from build123d import *

# Parameters (mm, degrees)
SKETCH1_R            = 12.5
BOSS_EXTRUDE1_DEPTH  = 4
BOSS_EXTRUDE7_DEPTH  = 4
SKETCH9_W            = 20
SKETCH9_H            = 36
BOSS_EXTRUDE8_DEPTH  = 4
BOSS_EXTRUDE9_DEPTH  = 8
BOSS_EXTRUDE10_DEPTH = 4
FILLET4_R            = 1
SKETCH11_R           = 2.5
CUT_EXTRUDE2_DEPTH   = 57.25989309
CHAMFER1_SIZE        = 10
SKETCH12_R           = 2.5
CUT_EXTRUDE3_DEPTH   = 4
FILLET5_R            = 1
SCALE1_SCALE         = 0.5


with BuildPart() as part:
    # Sketch1 → Boss-Extrude1 (new body)
    with BuildSketch(Plane.XY):
        Circle(SKETCH1_R)
        with BuildLine():
            Line((26.387505004, 12.5), (20, 12.5))
            Line((20, 12.5), (20, -12.5))
            Line((20, -12.5), (26.387505004, -12.5))
            ThreePointArc((26.387505004, -12.5), (22, 0), (26.387505004, 12.5))
        make_face()
        with BuildLine():
            Line((13.612494996, 12.5), (0, 12.5))
            ThreePointArc((0, 12.5), (8.838834765, 8.838834765), (12.5, 0))
            ThreePointArc((12.5, 0), (8.838834765, -8.838834765), (0, -12.5))
            Line((0, -12.5), (13.612494996, -12.5))
            ThreePointArc((13.612494996, -12.5), (18, 0), (13.612494996, 12.5))
        make_face()
        with BuildLine():
            Line((20, 12.5), (13.612494996, 12.5))
            ThreePointArc((13.612494996, 12.5), (18, 0), (13.612494996, -12.5))
            Line((13.612494996, -12.5), (20, -12.5))
            Line((20, -12.5), (20, 12.5))
        make_face()
    extrude(amount=BOSS_EXTRUDE1_DEPTH)

    # Sketch8 → Boss-Extrude7 (add)
    with BuildSketch(Plane(origin=(0, 0, 0), x_dir=(-1, 0, 0), z_dir=(0, 0, -1))):
        with BuildLine():
            Line((-26.387505004, 12.5), (-41.387505004, 12.5))
            Line((-41.387505004, 12.5), (-41.387505004, -12.5))
            Line((-41.387505004, -12.5), (-26.387505004, -12.5))
            ThreePointArc((-26.387505004, -12.5), (-22, 0), (-26.387505004, 12.5))
        make_face()
    extrude(amount=-BOSS_EXTRUDE7_DEPTH)


with BuildPart() as body_2:
    # Mirror3: mirrored copy
    add(part.part.mirror(Plane.XY.offset(18)))


with BuildPart() as part_1:
    add(part.part)

    add(body_2.part)  # Boss-Extrude8 merges body 2
    # Sketch9 → Boss-Extrude8 (add)
    with BuildSketch(Plane.XZ.offset(12.5)):
        with Locations((31.387505004, 18)):
            Rectangle(SKETCH9_W, SKETCH9_H)
    extrude(amount=-BOSS_EXTRUDE8_DEPTH)

    # Sketch1_4 → Boss-Extrude9 (add)
    with BuildSketch(Plane.XY):
        with BuildLine():
            Line((20, 12.5), (13.612494996, 12.5))
            ThreePointArc((13.612494996, 12.5), (18, 0), (13.612494996, -12.5))
            Line((13.612494996, -12.5), (20, -12.5))
            Line((20, -12.5), (20, 12.5))
        make_face()
        with BuildLine():
            Line((26.387505004, 12.5), (20, 12.5))
            Line((20, 12.5), (20, -12.5))
            Line((20, -12.5), (26.387505004, -12.5))
            ThreePointArc((26.387505004, -12.5), (22, 0), (26.387505004, 12.5))
        make_face()
        with BuildLine():
            Line((40, 12.5), (26.387505004, 12.5))
            ThreePointArc((26.387505004, 12.5), (22, 0), (26.387505004, -12.5))
            Line((26.387505004, -12.5), (40, -12.5))
            ThreePointArc((40, -12.5), (27.5, 0), (40, 12.5))
        make_face()
    boss_extrude9 = extrude(amount=BOSS_EXTRUDE9_DEPTH)

    # Sketch10 → Boss-Extrude10 (add)
    with BuildSketch(Plane.XY.offset(4)):
        with BuildLine():
            Line((41.387505004, 12.5), (40, 12.5))
            ThreePointArc((40, 12.5), (28.543560763, 5), (30.83484861, -8.5))
            Line((30.83484861, -8.5), (41.387505004, -8.5))
            Line((41.387505004, -8.5), (41.387505004, 12.5))
        make_face()
    boss_extrude10 = extrude(amount=BOSS_EXTRUDE10_DEPTH)

    # Mirror4: Boss-Extrude9, Boss-Extrude10 across plane
    add(boss_extrude9.mirror(Plane.XY.offset(18)))
    add(boss_extrude10.mirror(Plane.XY.offset(18)))

    # Fillet4
    fillet4_edges = [part_1.edges().sort_by_distance(p)[0] for p in [
        (13.612494996, -12.5, 30),
        (13.612494996, 12.5, 30),
        (13.612494996, -12.5, 6),
        (13.612494996, 12.5, 6),
    ]]
    fillet(fillet4_edges, radius=FILLET4_R)

    # Sketch11 → Cut-Extrude2 (cut, through all)
    with BuildSketch(Plane.XY.offset(36)):
        Circle(SKETCH11_R)
    extrude(amount=-CUT_EXTRUDE2_DEPTH, mode=Mode.SUBTRACT)

    # Chamfer1
    chamfer1_edges = [part_1.edges().sort_by_distance(p)[0] for p in [
        (41.387505004, 12.5, 4),
        (41.387505004, 12.5, 32),
    ]]
    chamfer(chamfer1_edges, length=CHAMFER1_SIZE)

    # Sketch12 → Cut-Extrude3 (cut)
    with BuildSketch(Plane(origin=(0, -8.5, 0), x_dir=(1, 0, 0), z_dir=(0, 1, 0))):
        with Locations(Location((32.387505004, -12, 0), (0, 0, 180))):
            Circle(SKETCH12_R)
        with Locations((32.387505004, -24)):
            Circle(SKETCH12_R)
    extrude(amount=-CUT_EXTRUDE3_DEPTH, mode=Mode.SUBTRACT)

    # Fillet5
    fillet5_edges = [part_1.edges().sort_by_distance(p)[0] for p in [
        (41.387505004, 2.5, 4),
        (41.387505004, 2.5, 32),
        (31.387505004, 12.5, 32),
        (31.387505004, 12.5, 4),
    ]]
    fillet(fillet5_edges, radius=FILLET5_R)


with BuildPart() as part_2:
    # Scale1: scaled about (0, 0, 0)
    add(part_1.part.scale(SCALE1_SCALE))


solid = part_2.part
Model file for the job. Use its own axes, mm. A direction names the side the tool comes from. Give positions to 0.01 mm unless a question says otherwise; leave off trailing zeros. Order: outer loops, then holes, each group sorted by start corner. A loop starts at its lowest first (then second) coordinate and runs counter-clockwise, first axis right, second up. Notation, with made-up numbers: (29, 25.5) - (80, 25.5) arc R14 ccw to (80, 44.5) - close; hole circle Ø6 at (-3.5, -15.5). An arc over 180 degrees is marked (long way). Write item = value, one per line. Start each with the question number.
1. Cut at A-A, the plane z = 6. List the corners of the cut face in (x, y).
2. Drop flat-ended pins along their axis: P1, Ø1.6, axis at y = -5.5, z = 10, coming from the -X side; P2, Ø3, axis at x = 16.19, z = 12, coming from the +Y side; P3, Ø5, axis at y = -3.5, z = 2.5, coming from the -X side. Give the stop position or say it passes through.
3. Cut at B-B, the plane z = 1.25. List the corners of the cut face in (x, y).
4. Which spindle directions (+Z, -Z, +X, -X, +Y, -Y) get a long thin tool onto all of the face, cutting with end or side? Do faces 5 (the flat face through (10.694, -5, 9)), 6 (the flat face through (18.161, 3.783, 2.028)), 7 (the cylindrical face through (9, 0, 15)). Say none if no direction does.
5. Cut at D-D, the plane y = 3.25. List the corners of the cut face in (x, z), and give its area (3 significant figures).
6. Probe line 1 along Z through (x, y) = (-3, -0.75); line 2 along X through (y, z) = (-5.8, 12); line 3 along Z through (x, y) = (18, -3.25). List the from-to ranges inside material, lowest first.
7. Two-plate mould, pull along Y, no slides. Class faces 1 (the flat face through (7, 0, 0)), 2 (the flat face through (16, -4.25, 9)), 3 (the cylindrical face through (9, 0, 3)), 4 (the cylindrical face through (-6.25, 0.14, 17.01)): pulls with the +Y half, pulls with the -Y half, needs draft (parallel to the pull), parting line crosses it, or undercut.
8. Cut at C-C, the plane x = 5. List the corners of the cut face in (y, z), and give its area (3 significant figures).
Taken from the geometry:
q1.outline = (10.69, -6.25) - (14.94, -6.25) - (14.94, -4.25) - (10.69, -4.25) - close; (17.44, -6.25) - (20.69, -6.25) - (20.69, -4.25) - (17.44, -4.25) - close
q2.P1 = 10.69
q2.P2 = -4.25
q2.P3 = -6.16
q3.outline = (0, -6.25) - (20.69, -6.25) - (20.69, 1.04) arc R0.5 ccw to (20.55, 1.4) - (15.84, 6.1) arc R0.5 ccw to (15.49, 6.25) - (0, 6.25) arc R6.25 ccw to start; hole circle Ø2.5 at (0, 0)
q4.face_5 = -X, +Y, -Y
q4.face_6 = +Z, -Z, +X, +Y
q4.face_7 = -X
q5.outline = (-5.34, 0) - (18.69, 0) - (18.69, 4) - (8.46, 4) - (8.46, 2) - (-5.34, 2) - close; (-5.34, 16) - (8.46, 16) - (8.46, 14) - (18.69, 14) - (18.69, 18) - (-5.34, 18) - close
q5.area = 137 mm²
q6.line_1 = 0 to 2, 16 to 18
q6.line_2 = 10.69 to 14.94, 17.44 to 20.69
q6.line_3 = 0 to 4, 14 to 18
q7.face_1 = needs draft
q7.face_2 = pulls with the +Y half
q7.face_3 = undercut
q7.face_4 = parting line crosses it
q8.outline = (-6.25, 0) - (6.25, 0) - (6.25, 2) - (-6.25, 2) - close; (-6.25, 16) - (6.25, 16) - (6.25, 18) - (-6.25, 18) - close
q8.area = 50.0 mm²
